Geometry check sheet. Reference: the model listing, model coordinates, mm. A direction names the side the tool comes from. Round coordinates to 2 decimals unless told otherwise and drop trailing zeros. Loops run counter-clockwise (first coordinate to the right, second up) from the corner with the lowest first, then second, coordinate; pieces in that order, holes last.
```python
from build123d import *

# Parameters (mm, degrees)
SKETCH1_R           = 5.715
BOSS_EXTRUDE1_DEPTH = 12.7
SKETCH3_R           = 5.715
BOSS_EXTRUDE2_DEPTH = 53.975
CUT_EXTRUDE1_DEPTH  = 53.975


with BuildPart() as part:
    # Sketch1 → Boss-Extrude1 (new body)
    with BuildSketch(Plane(origin=(0, 0, 0), x_dir=(1, 0, 0), z_dir=(0, 1, 0))):
        Circle(SKETCH1_R)
        with BuildLine():
            Line((1.905, -2.54), (-1.905, -2.54))
            ThreePointArc((-1.905, -2.54), (0, 3.175), (1.905, -2.54))
        make_face(mode=Mode.SUBTRACT)
    extrude(amount=BOSS_EXTRUDE1_DEPTH)

    # Sketch3 → Boss-Extrude2 (add)
    with BuildSketch(Plane(origin=(0, 0, 0), x_dir=(-1, 0, 0), z_dir=(0, -1, 0))):
        Circle(SKETCH3_R)
    extrude(amount=BOSS_EXTRUDE2_DEPTH)

    # Sketch4 → Cut-Extrude1 (cut)
    with BuildSketch(Plane.XZ.offset(53.975)):
        Polygon((0, 2.54), (-1.796051224, 4.336051224), (-4.336051224, 1.796051224), (-2.54, 0), (-4.336051224, -1.796051224), (-1.796051224, -4.336051224), (0, -2.54), (1.796051224, -4.336051224), (4.336051224, -1.796051224), (2.54, 0), (4.336051224, 1.796051224), (1.796051224, 4.336051224), align=None)
    extrude(amount=-CUT_EXTRUDE1_DEPTH, mode=Mode.SUBTRACT)


solid = part.part
```
1) Scan lines: line 1 along Z through (x, y) = (4, -40); line 2 along Z through (x, y) = (4.25, -21.5); line 3 along X through (y, z) = (9, 0) (3 decimals). Record each from-to range of solid material in increasing order.
Report:
line 1: z = -4.08 to -2.13, -1.46 to 1.46, 2.13 to 4.08
line 2: z = -3.82 to -1.88, -1.71 to 1.71, 1.88 to 3.82
line 3: x = -5.715 to -3.175, 3.175 to 5.715
2) Sectioned sample at B-B, the plane y = 4. Record the cut outline in (x, z) (3 decimals).
Report:
outline: circle Ø11.43 at (0, 0); hole (-1.905, 2.54) arc R3.175 ccw (long way) to (1.905, 2.54) - close
3) Sectioned sample at A-A, the plane y = -17. Record the cut outline in (x, z) (3 decimals).
Report:
outline: circle Ø11.43 at (0, 0); hole (-4.336, -1.796) - (-1.796, -4.336) - (0, -2.54) - (1.796, -4.336) - (4.336, -1.796) - (2.54, 0) - (4.336, 1.796) - (1.796, 4.336) - (0, 2.54) - (-1.796, 4.336) - (-4.336, 1.796) - (-2.54, 0) - close
4) Gauge pin test, flat ends, axial feed: pin 1 (0.7 mm diameter, centred on x = 0, z = -2.5, fed in from +Y); pin 2 (2 mm diameter, centred on y = -44, z = -1.5, fed in from +X). Record the tip position at first contact, or that the pin passes through.
Report:
pin 1: stops at y = 0
pin 2: stops at x = 5.69
5) Access from +Z, -Z, +X, -X, +Y, -Y to the whole of each face (thin tool, end or side, straight path). Record for faces 3 (the face through (2.5, 12.7, 2.5)), 4 (the face through (2, 0, 3)), 5 (the face through (-0.111, 6.261, -3.173)).
Report:
face 3: +Z, -Z, +X, -X, +Y
face 4: -Y
face 5: +Y
6) Mould release check, pull along Z, two halves, no side actions. Record for faces 1 (the face through (-2.6, 0, -2.6)), 2 (the face through (0, -53.975, 4)): +Z half, -Z half, draft (parallel to the pull), parting line (faces both ways), or undercut.
Report:
face 1: undercut
face 2: draft
